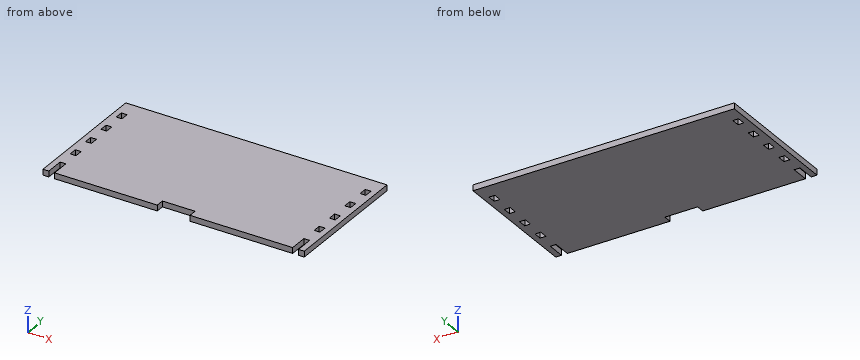
from build123d import *

# Parameters (mm, degrees)
SKETCH1_W           = 4.4958
SKETCH1_H           = 6.35
BOSS_EXTRUDE1_DEPTH = 4.4958
SKETCH2_W           = 25.4
SKETCH2_H           = 6.35
CUT_EXTRUDE1_DEPTH  = 228.799668827


with BuildPart() as part:
    # Sketch1 → Boss-Extrude1 (new body)
    with BuildSketch(Plane.XY):
        Polygon((0, 102.87), (0, 0), (4.5085, 0), (4.5085, 7.62), (4.5085, 13.97), (9.0043, 13.97), (9.0043, 7.62), (9.0043, 0), (194.1957, 0), (194.1957, 7.62), (194.1957, 13.97), (198.6915, 13.97), (198.6915, 7.62), (198.6915, 0), (203.2, 0), (203.2, 102.87), align=None)
        with Locations((6.7564, 29.845)):
            Rectangle(SKETCH1_W, SKETCH1_H, mode=Mode.SUBTRACT)
        with Locations((6.7564, 48.895)):
            Rectangle(SKETCH1_W, SKETCH1_H, mode=Mode.SUBTRACT)
        with Locations((196.4436, 29.845)):
            Rectangle(SKETCH1_W, SKETCH1_H, mode=Mode.SUBTRACT)
        with Locations((196.4436, 48.895)):
            Rectangle(SKETCH1_W, SKETCH1_H, mode=Mode.SUBTRACT)
        with Locations((6.7564, 67.945)):
            Rectangle(SKETCH1_W, SKETCH1_H, mode=Mode.SUBTRACT)
        with Locations((6.7564, 86.995)):
            Rectangle(SKETCH1_W, SKETCH1_H, mode=Mode.SUBTRACT)
        with Locations((196.4436, 67.945)):
            Rectangle(SKETCH1_W, SKETCH1_H, mode=Mode.SUBTRACT)
        with Locations((196.4436, 86.995)):
            Rectangle(SKETCH1_W, SKETCH1_H, mode=Mode.SUBTRACT)
    extrude(amount=BOSS_EXTRUDE1_DEPTH)

    # Sketch2 → Cut-Extrude1 (cut, through all)
    with BuildSketch(Plane.XY.offset(4.4958)):
        with Locations((101.6, 3.175)):
            Rectangle(SKETCH2_W, SKETCH2_H)
    extrude(amount=-CUT_EXTRUDE1_DEPTH, mode=Mode.SUBTRACT)


solid = part.part
Design review of the part built by this model. Coordinates are the model's own, in mm. Coordinates: 2 decimals unless noted, no trailing zeros. Loops run counter-clockwise (first coordinate to the right, second up) from the corner with the lowest first, then second, coordinate; pieces in that order, holes last. Notation, with made-up numbers: M 76.25,13 L 85.25,13 A11 ccw 85.25,23 Z; hole C 51.5,10 d4. An arc over 180 degrees is marked long. Use one line per item in the form item = value.
(1) Consider section B-B (z = 1.35). Give the number of separate pieces and of enclosed holes in the cut face, and give its area (3 significant figures).
Return value:
separate_pieces = 1
enclosed_holes = 8
area = 20,400 mm2
(2) Consider section A-A (y = 49). Write out the cut boundary in (x, z), and give its area (3 significant figures).
Return value:
outline = M 0,0 L 4.51,0 L 4.51,4.5 L 0,4.5 Z; M 9,0 L 194.2,0 L 194.2,4.5 L 9,4.5 Z; M 198.69,0 L 203.2,0 L 203.2,4.5 L 198.69,4.5 Z
area = 873 mm2
(3) Consider section C-C (x = 108). Write out the cut boundary in (y, z).
Return value:
outline = M 6.35,0 L 102.87,0 L 102.87,4.5 L 6.35,4.5 Z
(4) Clearance check with a flat-ended pin moving along its axis: P1, Ø2, axis at x = 196.5, z = 2.5, coming from the -Y side. State where the tip first meets the part, or that it passes through.
Return value:
P1 = 13.97
(5) For line 1 along X through (y, z) = (71, 3.6); line 2 along Y through (x, z) = (98, 3.45), list the stretches that pass through material, from the lowest coordinate up. Write a range as from..to.
Return value:
line_1 = 0..4.51, 9..194.2, 198.69..203.2
line_2 = 6.35..102.87
